Can you work these out from the model? Positions are in its coordinate system, mm. A direction names the side the tool comes from. Round coordinates to 2 decimals unless told otherwise and drop trailing zeros. Loops run counter-clockwise (first coordinate to the right, second up) from the corner with the lowest first, then second, coordinate; pieces in that order, holes last.
(1) I want a section at D-D on z = 23. Write out the boundary of the cut face in (x, y), plus the area to 3 significant figures.
(2) I want a section at B-B on x = 0. Write out the boundary of the cut face in (y, z).
(3) I want a section at A-A on z = 5. Write out the boundary of the cut face in (x, y), plus the area to 3 significant figures.
(4) If I drill on line 1 along X through (y, z) = (9.5, 10.5); line 2 along Y through (x, z) = (0, 9.5); line 3 along Y through (x, z) = (-5.75, 9.75), over which ranges is the centre line in solid material (lowest first)?
(5) Will these pins go through, and if not, where does the flat tip stop? pin 1 Ø5 at (x, z) = (-10.32, 25) entering from +Y; pin 2 Ø6 at (x, z) = (7.5, 16.5) entering from +Y; pin 3 Ø6 at (y, z) = (7.5, 14) entering from -X.
(6) Thinking about a two-plate mould opening in X: for faces 1 (the face through (-10, 2.8, 15)), 2 (the face through (0.08, 13.05, 14.79)), 3 (the face through (10.513, 1.42, 26.487)), which applies, released by +X, released by -X, zero draft, split by the parting line, or undercut?
(7) Which directions (+Z, -Z, +X, -X, +Y, -Y) give clear straight access to the entire face, cutting with the end or side of a thin tool? Please do faces 4 (the face through (0, 4, 0)), 5 (the face through (10, 2.8, 15)).
(8) I want a section at C-C on x = 10.25. Write out the boundary of the cut face in (y, z), plus the area to 3 significant figures.
from build123d import *

# Parameters (mm, degrees)
F0_R     = 1.35
F1_DEPTH = 30
F2_R     = 3
F3_R     = 1.5
F4_DEPTH = 25


with BuildPart() as f1:
    # F0 (on Top) → F1 (new body)
    with BuildSketch(Plane.XY):
        with BuildLine():
            ThreePointArc((-3.0028277119, 7.4646546511), (0, 5.85036), (3.0028277119, 7.4646546511))
            Line((3.0028277119, 7.4646546511), (3.6, 9.45036))
            ThreePointArc((3.6, 9.45036), (0, 13.05036), (-3.6, 9.45036))
            Line((-3.6, 9.45036), (-3.0028277119, 7.4646546511))
        make_face()
        with Locations((0, 9.45036)):
            Circle(F0_R, mode=Mode.SUBTRACT)
        with BuildLine():
            Line((-1.6, 2.8), (1.6, 2.8))
            Line((1.6, 2.8), (3.0028277119, 7.4646546511))
            ThreePointArc((3.0028277119, 7.4646546511), (0, 5.85036), (-3.0028277119, 7.4646546511))
            Line((-3.0028277119, 7.4646546511), (-1.6, 2.8))
        make_face()
        Polygon((-15, 0), (15, 0), (15, 2.8), (1.6, 2.8), (-1.6, 2.8), (-15, 2.8), align=None)
    extrude(amount=F1_DEPTH)

    # F2
    f2_edges = [f1.edges().sort_by_distance(p)[0] for p in [
        (-1.6, 2.8, 15),
        (1.6, 2.8, 15),
    ]]
    fillet(f2_edges, radius=F2_R)

    # F3 (on face) → F4 (cut)
    with BuildSketch(Plane(origin=(0, 2.8, 0), x_dir=(-1, 0, 0), z_dir=(0, 1, 0))):
        with Locations((-10.3174667911, 25)):
            Circle(F3_R)
        with Locations((-10.3174667911, 5)):
            Circle(F3_R)
        with Locations((10.31747, 5)):
            Circle(F3_R)
        with Locations((10.31747, 25)):
            Circle(F3_R)
    extrude(amount=-F4_DEPTH, mode=Mode.SUBTRACT)


solid = f1.part
Filled sheet:
1. outline: (-15, 0) - (15, 0) - (15, 2.8) - (5.63, 2.8) arc R3 cw to (2.76, 6.66) - (3.6, 9.45) arc R3.6 ccw to (-3.6, 9.45) - (-2.76, 6.66) arc R3 cw to (-5.63, 2.8) - (-15, 2.8) - close; hole circle Ø2.7 at (0, 9.45)
1. area: 141 mm2
2. outline: (0, 0) - (8.1, 0) - (8.1, 30) - (0, 30) - close; (10.8, 0) - (13.05, 0) - (13.05, 30) - (10.8, 30) - close
3. outline: (-15, 0) - (-11.82, 0) - (-11.82, 2.8) - (-15, 2.8) - close; (-8.82, 0) - (8.82, 0) - (8.82, 2.8) - (5.63, 2.8) arc R3 cw to (2.76, 6.66) - (3.6, 9.45) arc R3.6 ccw to (-3.6, 9.45) - (-2.76, 6.66) arc R3 cw to (-5.63, 2.8) - (-8.82, 2.8) - close; (11.82, 0) - (15, 0) - (15, 2.8) - (11.82, 2.8) - close; hole circle Ø2.7 at (0, 9.45)
3. area: 124 mm2
4. line 1: x = -3.6 to -1.35, 1.35 to 3.6
4. line 2: y = 0 to 8.1, 10.8 to 13.05
4. line 3: y = 0 to 2.8
5. pin 1: stops at y = 2.8
5. pin 2: stops at y = 3.02
5. pin 3: stops at x = -3.6
6. face 1: zero draft
6. face 2: split by the parting line
6. face 3: undercut
7. face 4: -Z, +X, -X, +Y, -Y
7. face 5: +Z, -Z, +X, +Y
8. outline: (0, 0) - (2.8, 0) - (2.8, 3.5) - (0, 3.5) - close; (0, 6.5) - (2.8, 6.5) - (2.8, 23.5) - (0, 23.5) - close; (0, 26.5) - (2.8, 26.5) - (2.8, 30) - (0, 30) - close
8. area: 67.2 mm2
